```python
from build123d import *

# Parameters (mm, degrees)
HEAD_SKETCH_R                  = 2.25
HEAD_DEPTH                     = 2
THREADED_SECTION_STUB_SKETCH_R = 1.5
BOSS_EXTRUDE2_DEPTH            = 5
END_OF_BOLT_CHAMFER_SIZE       = 0.5
END_OF_BOLT_CHAMFER_SIZE2      = 0.288675135
COSMETIC_FILLETS_R             = 0.2


with BuildPart() as part:
    # Head Sketch → Head (new body)
    with BuildSketch(Plane(origin=(0, 0, 0), x_dir=(1, 0, 0), z_dir=(0, 1, 0))):
        with Locations(Location((0, 0, 0), (0, 0, 270))):
            Circle(HEAD_SKETCH_R)
        Polygon((-0.577350269, 1), (-1.154700538, 0), (-0.577350269, -1), (0.577350269, -1), (1.154700538, 0), (0.577350269, 1), align=None, mode=Mode.SUBTRACT)
    extrude(amount=HEAD_DEPTH)

    # Threaded Section Stub Sketch → Boss-Extrude2 (add)
    with BuildSketch(Plane(origin=(0, 0, 0), x_dir=(1, 0, 0), z_dir=(0, 1, 0))):
        with Locations(Location((0, 0, 0), (0, 0, 270))):
            Circle(THREADED_SECTION_STUB_SKETCH_R)
    extrude(amount=-BOSS_EXTRUDE2_DEPTH)

    # End Of Bolt chamfer
    end_of_bolt_chamfer_edges = [part.edges().sort_by_distance(p)[0] for p in [
        (0, -5, -1.5),
    ]]
    end_of_bolt_chamfer_side = [part.faces().sort_by_distance(p)[0] for p in [
        (0, -5, 0),
    ]]
    chamfer(end_of_bolt_chamfer_edges, length=END_OF_BOLT_CHAMFER_SIZE, length2=END_OF_BOLT_CHAMFER_SIZE2, reference=end_of_bolt_chamfer_side[0])

    # Cosmetic Fillets
    cosmetic_fillets_edges = [part.edges().sort_by_distance(p)[0] for p in [
        (-0.577350269, 1, -1),
        (-0.8660254037844384, 0, 0.5000000000000003),
        (-1.154700538, 1, 0),
        (0, 0, 1),
        (-0.577350269, 1, 1),
        (0.8660254037844388, 0, 0.4999999999999998),
        (0.577350269, 1, 1),
        (0.8660254037844388, 0, -0.5000000000000002),
        (0, 2, -1),
        (-0.866025404, 2, -0.5),
        (-0.866025404, 2, 0.5),
        (0, 2, 1),
        (0.866025404, 2, 0.5),
        (0.866025404, 2, -0.5),
        (0, 0, -2.25),
        (0, 2, -2.25),
        (0, 0, -1),
        (0.577350269, 1, -1),
        (-0.8660254037844386, 0, -0.4999999999999998),
    ]]
    fillet(cosmetic_fillets_edges, radius=COSMETIC_FILLETS_R)


solid = part.part
```
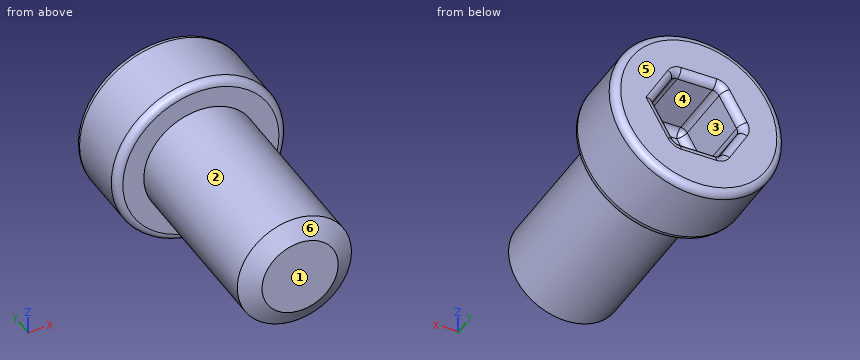
Geometry: final body of the model. Coordinates: model frame, mm. Face numbers are marked on the shaded views. A direction names the side the tool comes from. Coordinates: 2 decimals unless noted, no trailing zeros. Order: outer loops, then holes, each group sorted by start corner. A loop starts at its lowest first (then second) coordinate and runs counter-clockwise, first axis right, second up.
Item 1: Section query B-B (y = -4.25). Output: boundary loops of the cut face in (x, z), then the cut area to 3 significant figures.
Answer:
outline: circle Ø3 at (0, 0)
area: 7.07 mm2
Item 2: Access query for the marked faces 1, 2 and 3. Directions: +Z, -Z, +X, -X, +Y, -Y. A direction counts if a zero-diameter tool reaches every point of the face in a straight line with its end or side. Return the directions, or none.
Answer:
face 1: +Z, -Z, +X, -X, -Y
face 2: -Y
face 3: +Y
Item 3: Section query A-A (y = 1). Output: boundary loops of the cut face in (x, z).
Answer:
outline: circle Ø4.5 at (0, 0); hole (-1.1, -0.1) - (-0.64, -0.9) arc R0.2 ccw to (-0.46, -1) - (0.46, -1) arc R0.2 ccw to (0.64, -0.9) - (1.15, 0) - (0.64, 0.9) arc R0.2 ccw to (0.46, 1) - (-0.46, 1) arc R0.2 ccw to (-0.64, 0.9) - (-1.1, 0.1) arc R0.2 ccw to start
Item 4: Draft query along X for the marked faces 4, 5 and 6. Return one class per face: released by +X, released by -X, zero draft, split by the parting line, or undercut.
Answer:
face 4: undercut
face 5: zero draft
face 6: split by the parting line
Item 5: Material intervals for line 1 along Y through (x, z) = (1.15, 1.25); line 2 along Z through (x, y) = (-1, 0.5); line 3 along X through (y, z) = (0.25, -0.5), sorted ascending.
Answer:
line 1: y = 0 to 2
line 2: z = -2.02 to -0.27, 0.27 to 2.02
line 3: x = -2.19 to -0.87, 0.87 to 2.19
Item 6: Contact query for flat-ended pins moving along their axis: P1, Ø1.5, axis at x = 1.5, z = 1, coming from the -Y side; P2, Ø1, axis at y = -2, z = 0.5, coming from the -X side; P3, Ø0.8, axis at x = 0.5, z = 0, coming from the +Y side. Output: stop coordinate, or through.
Answer:
P1: stops at y = -4.97
P2: stops at x = -1.5
P3: stops at y = 0
